Model file for the job. Use its own axes, mm. A direction names the side the tool comes from. Round coordinates to 2 decimals unless told otherwise and drop trailing zeros. Order: outer loops, then holes, each group sorted by start corner. A loop starts at its lowest first (then second) coordinate and runs counter-clockwise, first axis right, second up. Notation, with made-up numbers: (35.5, 12) - (72.5, 12) arc R23 cw to (72.5, 34) - close; hole circle Ø6 at (78.5, -18). An arc over 180 degrees is marked (long way). Write item = value, one per line. Start each with the question number.
from build123d import *

# Parameters (mm, degrees)
CROQUIS1_R              = 19
SALIENTE_EXTRUIR1_DEPTH = 5
CORTAR_EXTRUIR1_DEPTH   = 3.6
CROQUIS6_R              = 2.25
CORTAR_EXTRUIR2_DEPTH   = 10


with BuildPart() as part:
    # Croquis1 → Saliente-Extruir1 (new, symmetric)
    with BuildSketch(Plane.XY):
        with BuildLine():
            Line((-29, 19.595917942), (-29, 35))
            Line((-29, 35), (29, 35))
            Line((29, 35), (29, 19.595917942))
            ThreePointArc((29, 19.595917942), (35, 0), (29, -19.595917942))
            Line((29, -19.595917942), (29, -35))
            Line((29, -35), (-29, -35))
            Line((-29, -35), (-29, -19.595917942))
            ThreePointArc((-29, -19.595917942), (-35, 0), (-29, 19.595917942))
        make_face()
        Circle(CROQUIS1_R, mode=Mode.SUBTRACT)
    extrude(amount=SALIENTE_EXTRUIR1_DEPTH, both=True)

    # Croquis5 → Cortar-Extruir1 (cut)
    with BuildSketch(Plane(origin=(0, 28, 0), x_dir=(1, 0, 0), z_dir=(0, 1, 0))):
        Polygon((-23.7, -2.136195996), (-23.7, -5), (-16.3, -5), (-16.3, -2.136195996), (-16.3, 2.136195996), (-20, 4.272391992), (-23.7, 2.136195996), align=None)
        Polygon((16.3, 2.136195996), (16.3, -2.136195996), (16.3, -5), (23.7, -5), (23.7, -2.136195996), (23.7, 2.136195996), (20, 4.272391992), align=None)
    cortar_extruir1 = extrude(amount=CORTAR_EXTRUIR1_DEPTH, mode=Mode.SUBTRACT)

    # Croquis6 → Cortar-Extruir2 (cut)
    with BuildSketch(Plane(origin=(0, 35, 0), x_dir=(1, 0, 0), z_dir=(0, 1, 0))):
        with Locations(Location((-20, 0, 0), (0, 0, 270))):
            Circle(CROQUIS6_R)
        with Locations(Location((20, 0, 0), (0, 0, 270))):
            Circle(CROQUIS6_R)
    cortar_extruir2 = extrude(amount=-CORTAR_EXTRUIR2_DEPTH, mode=Mode.SUBTRACT)

    # Simetría1: Cortar-Extruir1, Cortar-Extruir2 across plane
    add(cortar_extruir1.mirror(Plane.ZX), mode=Mode.SUBTRACT)
    add(cortar_extruir2.mirror(Plane.ZX), mode=Mode.SUBTRACT)


solid = part.part
Item 1: Saw through at C-C, the plane y = -27. Give the cut face in (x, z).
Item 2: Mould opens along Y. For faces 1 (the face through (-20.1, -28, 2.4)), 2 (the face through (-20, -25, 0)), 3 (the face through (-29, 27, 0)) say: +Y half, -Y half, draft (parallel to the pull), parting line (faces both ways), or undercut.
Item 3: Saw through at A-A, the plane x = 0. Give the cut face in (y, z), then the cut area to 3 significant figures.
Item 4: Probe L1, parallel to X at y = 33.95, z = 0; L2, parallel to Y at x = 21.5, z = 3.5; L3, parallel to X at y = -29.5, z = 4.25. List the from-to ranges inside material, lowest first.
Item 5: Saw through at B-B, the plane y = 15. Give the cut face in (x, z).
Item 6: Drop flat-ended pins along their axis: pin 1 (3.5 mm diameter, centred on x = 19.5, z = -0.5, fed in from -Y); pin 2 (4 mm diameter, centred on y = -30, z = 0, fed in from -X); pin 3 (3 mm diameter, centred on y = -30.5, z = 2.5, fed in from +X); pin 4 (2 mm diameter, centred on y = 5.5, z = -2.5, fed in from -X). Give the stop position or say it passes through.
Item 7: Which spindle directions (+Z, -Z, +X, -X, +Y, -Y) get a long thin tool onto all of the face, cutting with end or side? Do faces 4 (the face through (17.804, 26.521, -0.488)), 5 (the face through (-20.1, 28, 2.4)), 6 (the face through (-15, 16, 5)). Say none if no direction does.
Check sheet entries:
q1.outline = (-29, -5) - (29, -5) - (29, 5) - (-29, 5) - close; hole circle Ø4.5 at (-20, 0); hole circle Ø4.5 at (20, 0)
q2.face_1 = undercut
q2.face_2 = -Y half
q2.face_3 = draft
q3.outline = (-35, -5) - (-19, -5) - (-19, 5) - (-35, 5) - close; (19, -5) - (35, -5) - (35, 5) - (19, 5) - close
q3.area = 320 mm2
q4.L1 = -29 to -22.25, -17.75 to 17.75, 22.25 to 29
q4.L2 = -35 to -31.6, -28 to 28, 31.6 to 35
q4.L3 = -29 to -23.7, -16.3 to 16.3, 23.7 to 29
q5.outline = (-31.62, -5) - (-11.66, -5) - (-11.66, 5) - (-31.62, 5) - close; (11.66, -5) - (31.62, -5) - (31.62, 5) - (11.66, 5) - close
q6.pin_1 = -35
q6.pin_2 = -29
q6.pin_3 = 29
q6.pin_4 = -34.71
q7.face_4 = +Y
q7.face_5 = +Z
q7.face_6 = +Z, +X, -X, +Y, -Y
